Could you check a few things on this model? Use its own coordinates, in mm. Face numbers are marked on the shaded views. A direction names the side the tool comes from. Coordinates: 2 decimals unless noted, no trailing zeros. Loops run counter-clockwise (first coordinate to the right, second up) from the corner with the lowest first, then second, coordinate; pieces in that order, holes last. Notation, with made-up numbers: (-19, -1.75) -> (-11, -1.75) arc R19 cw to (-11, 14.25) -> close; hole circle Ø7 at (67, -18). An arc over 180 degrees is marked (long way). One line per question, with ' | ' between items. Start each with the question number.
(1) Suppose I cut it at C-C (x = 0). Please give me the cut outline in (y, z), plus the area to 3 significant figures.
(2) I'm going to push flat-ended pins straight in: pin 1 Ø0.8 at (y, z) = (-1.5, 2) entering from -X; pin 2 Ø0.8 at (x, z) = (1.5, 1.5) entering from -Y; pin 3 Ø0.5 at (y, z) = (-1.5, 1.5) entering from +X. Where does each tip first touch, or does it pass through?
(3) Suppose I cut it at A-A (z = -1.5). Please give me the cut outline in (x, y), plus the area to 3 significant figures.
(4) If I drill on line 1 along Z through (x, y) = (-6.25, 5); line 2 along Y through (x, z) = (0, 0.25); line 3 along Y through (x, z) = (-0.5, -3), over which ranges is the centre line in solid material (lowest first)?
(5) Suppose I cut it at B-B (y = 0). Please give me the cut outline in (x, z).
(6) Which directions (+Z, -Z, +X, -X, +Y, -Y) give clear straight access to the entire face, cutting with the end or side of a thin tool? Please do the marked faces 1 and 2.
(7) Suppose I cut it at D-D (y = -3.25). Please give me the cut outline in (x, z), plus the area to 3 significant figures.
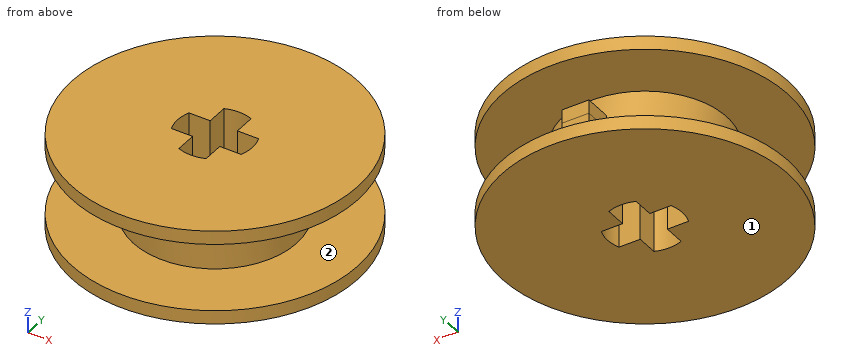
```python
from build123d import *

# Parameters (mm, degrees)
ESQUISSE1_R        = 6
BOSS_EXTRU_1_DEPTH = 2.5
ESQUISSE2_R        = 10.5
BOSS_EXTRU_4_DEPTH = 1
ESQUISSE3_W        = 2
ESQUISSE3_H        = 2
BOSS_EXTRU_5_DEPTH = 1


with BuildPart() as part:
    # Esquisse1 → Boss.-Extru.1 (new body)
    with BuildSketch(Plane.XY):
        Circle(ESQUISSE1_R)
        with BuildLine():
            Line((-2.561737691, 1), (-1, 1))
            Line((-1, 1), (-1, 2.561737691))
            ThreePointArc((-1, 2.561737691), (0, 2.75), (1, 2.561737691))
            Line((1, 2.561737691), (1, 1))
            Line((1, 1), (2.561737691, 1))
            ThreePointArc((2.561737691, 1), (2.75, 0), (2.561737691, -1))
            Line((2.561737691, -1), (1, -1))
            Line((1, -1), (1, -2.561737691))
            ThreePointArc((1, -2.561737691), (0, -2.75), (-1, -2.561737691))
            Line((-1, -2.561737691), (-1, -1))
            Line((-1, -1), (-2.561737691, -1))
            ThreePointArc((-2.561737691, -1), (-2.75, 0), (-2.561737691, 1))
        make_face(mode=Mode.SUBTRACT)
    boss_extru_1 = extrude(amount=BOSS_EXTRU_1_DEPTH)

    # Esquisse2 → Boss.-Extru.4 (add)
    with BuildSketch(Plane.XY.offset(2.5)):
        Circle(ESQUISSE2_R)
        with BuildLine():
            Line((-1, 2.561737691), (-1, 1))
            Line((-1, 1), (-2.561737691, 1))
            ThreePointArc((-2.561737691, 1), (-2.75, 0), (-2.561737691, -1))
            Line((-2.561737691, -1), (-1, -1))
            Line((-1, -1), (-1, -2.561737691))
            ThreePointArc((-1, -2.561737691), (0, -2.75), (1, -2.561737691))
            Line((1, -2.561737691), (1, -1))
            Line((1, -1), (2.561737691, -1))
            ThreePointArc((2.561737691, -1), (2.75, 0), (2.561737691, 1))
            Line((2.561737691, 1), (1, 1))
            Line((1, 1), (1, 2.561737691))
            ThreePointArc((1, 2.561737691), (0, 2.75), (-1, 2.561737691))
        make_face(mode=Mode.SUBTRACT)
    boss_extru_4 = extrude(amount=BOSS_EXTRU_4_DEPTH)

    # Esquisse3 → Boss.-Extru.5 (add)
    with BuildSketch(Plane(origin=(0, 0, 0), x_dir=(-1, 0, 0), z_dir=(0, 0, -1))):
        with Locations((0, 6.916079783)):
            Rectangle(ESQUISSE3_W, ESQUISSE3_H)
    boss_extru_5 = extrude(amount=-BOSS_EXTRU_5_DEPTH)


with BuildPart() as sym_trie1_1:
    # Symétrie1: Boss.-Extru.1, Boss.-Extru.4, Boss.-Extru.5 across Front Plane
    add(boss_extru_1.mirror(Plane.XY))
    add(boss_extru_4.mirror(Plane.XY))
    add(boss_extru_5.mirror(Plane.XY))


with BuildPart() as part_1:
    add(part.part)

    # Symétrie1 united with what the copies to: union Symétrie1_1
    add(sym_trie1_1.part)


solid = part_1.part
```
Checks:
1) outline: (-10.5, -3.5) -> (-2.75, -3.5) -> (-2.75, 3.5) -> (-10.5, 3.5) -> (-10.5, 2.5) -> (-6, 2.5) -> (-6, -2.5) -> (-10.5, -2.5) -> close; (2.75, -3.5) -> (10.5, -3.5) -> (10.5, -2.5) -> (6, -2.5) -> (6, -1) -> (7.92, -1) -> (7.92, 1) -> (6, 1) -> (6, 2.5) -> (10.5, 2.5) -> (10.5, 3.5) -> (2.75, 3.5) -> close | area: 67.3 mm^2
2) pin 1: stops at x = -5.9 | pin 2: stops at y = -5.9 | pin 3: stops at x = 5.87
3) outline: circle Ø12 at (0, 0); hole (-2.56, -1) -> (-1, -1) -> (-1, -2.56) arc R2.75 ccw to (1, -2.56) -> (1, -1) -> (2.56, -1) arc R2.75 ccw to (2.56, 1) -> (1, 1) -> (1, 2.56) arc R2.75 ccw to (-1, 2.56) -> (-1, 1) -> (-2.56, 1) arc R2.75 ccw to start | area: 95.6 mm^2
4) line 1: z = -3.5 to -2.5, 2.5 to 3.5 | line 2: y = -6 to -2.75, 2.75 to 7.92 | line 3: y = -10.49 to -2.7, 2.7 to 10.49
5) outline: (-10.5, -3.5) -> (-2.75, -3.5) -> (-2.75, 3.5) -> (-10.5, 3.5) -> (-10.5, 2.5) -> (-6, 2.5) -> (-6, -2.5) -> (-10.5, -2.5) -> close; (2.75, -3.5) -> (10.5, -3.5) -> (10.5, -2.5) -> (6, -2.5) -> (6, 2.5) -> (10.5, 2.5) -> (10.5, 3.5) -> (2.75, 3.5) -> close
6) face 1: -Z, +X, -X, +Y, -Y | face 2: none
7) outline: (-9.98, -3.5) -> (9.98, -3.5) -> (9.98, -2.5) -> (5.04, -2.5) -> (5.04, 2.5) -> (9.98, 2.5) -> (9.98, 3.5) -> (-9.98, 3.5) -> (-9.98, 2.5) -> (-5.04, 2.5) -> (-5.04, -2.5) -> (-9.98, -2.5) -> close | area: 90.4 mm^2
